Geometry check sheet. Reference: the model listing, model coordinates, mm. Face numbers are marked on the shaded views. A direction names the side the tool comes from. Round coordinates to 2 decimals unless told otherwise and drop trailing zeros. Loops run counter-clockwise (first coordinate to the right, second up) from the corner with the lowest first, then second, coordinate; pieces in that order, holes last. Notation, with made-up numbers: (41, 17) - (73, 17) arc R15 cw to (73, 27) - close; hole circle Ø1 at (79.25, 52.5). An arc over 180 degrees is marked (long way). Answer in a Markdown table with one row per item. Add a question column.
```python
from build123d import *
from build123d.topology import SkipClean

# Parameters (mm, degrees)
SKETCH_1_W                     = 41
SKETCH_1_H                     = 50
EXTRUDE_1_DEPTH                = 3
SKETCH_3_W                     = 15.5
SKETCH_3_H                     = 22
CUT_EXTRUDE_1_DEPTH            = 18
HOLE_WIZARD_M3_5_1_D           = 3.15
HOLE_WIZARD_M3_5_1_CSINK_D     = 3.55
HOLE_WIZARD_M3_5_1_CSINK_ANGLE = 90
SKETCH_16_W                    = 41
SKETCH_16_H                    = 0.872109694
EXTRUDE_5_DEPTH                = 20
SKETCH_17_W                    = 41
SKETCH_17_H                    = 50
SKETCH_17_R                    = 1.575
EXTRUDE_6_DEPTH                = 3
SKETCH_20_W                    = 26
SKETCH_20_H                    = 50
EXTRUDE_8_DEPTH                = 2
SKETCH_21_W                    = 12
SKETCH_21_H                    = 25
CUT_EXTRUDE_2_DEPTH            = 2
SKETCH_22_W                    = 26
SKETCH_22_H                    = 50
EXTRUDE_9_DEPTH                = 2
SKETCH_27_W                    = 20
SKETCH_27_H                    = 25
CUT_EXTRUDE_3_DEPTH            = 2
HOLE_WIZARD_M3_5_2_D           = 2.9
HOLE_WIZARD_M3_5_2_DEPTH       = 10
HOLE_WIZARD_M3_5_2_CSINK_D     = 3.55
HOLE_WIZARD_M3_5_2_CSINK_ANGLE = 90
HOLE_WIZARD_M3_5_2_TIP         = 0.871247898
SKETCH_36_R                    = 2.218303603
SKETCH_36_R_2                  = 1.575
SKETCH_36_R_3                  = 2.18160311
SKETCH_36_R_4                  = 2.164555566
SKETCH_36_R_5                  = 1.714538104
EXTRUDE_10_DEPTH               = 1
EXTRUDE_START                  = 1
SKETCH_37_R                    = 2.094490393
SKETCH_37_R_2                  = 1.575
SKETCH_37_R_3                  = 1.99590809
SKETCH_37_R_4                  = 2.064181582
EXTRUDE_11_DEPTH               = 1
SKETCH_38_R                    = 2.007165216
SKETCH_38_R_2                  = 1.775
SKETCH_38_R_3                  = 2.052187766
SKETCH_38_R_4                  = 2.157504148
SKETCH_38_R_5                  = 2.13214376
EXTRUDE_12_DEPTH               = 0.5


with BuildPart() as part:
    # Sketch 1 → Extrude 1 (new body)
    with BuildSketch(Plane.XY):
        Rectangle(SKETCH_1_W, SKETCH_1_H)
    extrude(amount=EXTRUDE_1_DEPTH)

    # Sketch 3 → Cut-Extrude 1 (cut)
    with BuildSketch(Plane.XY.offset(3)):
        with Locations((0, 14)):
            Rectangle(SKETCH_3_W, SKETCH_3_H)
    extrude(amount=-CUT_EXTRUDE_1_DEPTH, mode=Mode.SUBTRACT)

    # Hole Wizard M3.5 _ _1 (through all)
    with Locations(Plane.XY.offset(3)):
        with Locations((-3.5, -19), (3.5, -19), (-15.5, -11)):
            CounterSinkHole(HOLE_WIZARD_M3_5_1_D / 2, HOLE_WIZARD_M3_5_1_CSINK_D / 2, counter_sink_angle=HOLE_WIZARD_M3_5_1_CSINK_ANGLE)

    # Sketch 16 → Extrude 5 (add)
    with BuildSketch(Plane(origin=(0, 0, 0), x_dir=(-1, 0, 0), z_dir=(0, 0, -1))):
        with Locations((0, -24.563945153)):
            Rectangle(SKETCH_16_W, SKETCH_16_H)
    extrude(amount=EXTRUDE_5_DEPTH)



with BuildPart() as body_2:
    # Sketch 17 → Extrude 6 (new body)
    with BuildSketch(Plane(origin=(0, 0, -20), x_dir=(-1, 0, 0), z_dir=(0, 0, -1))):
        Rectangle(SKETCH_17_W, SKETCH_17_H)
        with Locations(Location((15.5, -11, 0), (0, 0, 180))):
            Circle(SKETCH_17_R, mode=Mode.SUBTRACT)
        with Locations(Location((3.5, -19, 0), (0, 0, 180))):
            Circle(SKETCH_17_R, mode=Mode.SUBTRACT)
        with Locations(Location((-3.5, -19, 0), (0, 0, 180))):
            Circle(SKETCH_17_R, mode=Mode.SUBTRACT)
    extrude(amount=EXTRUDE_6_DEPTH)


with BuildPart() as part_1:
    add(part.part)

    add(body_2.part)  # Extrude 8 merges body 2
    # Sketch 20 → Extrude 8 (add)
    with BuildSketch(Plane(origin=(20.5, 0, 0), x_dir=(0, 0, -1), z_dir=(1, 0, 0))):
        with Locations((10, 0)):
            Rectangle(SKETCH_20_W, SKETCH_20_H)
    extrude(amount=EXTRUDE_8_DEPTH)

    # Sketch 21 → Cut-Extrude 2 (cut)
    with BuildSketch(Plane(origin=(22.5, 0, 0), x_dir=(0, 0, -1), z_dir=(1, 0, 0))):
        with Locations((6, 12.5)):
            Rectangle(SKETCH_21_W, SKETCH_21_H)
    extrude(amount=-CUT_EXTRUDE_2_DEPTH, mode=Mode.SUBTRACT)

    # Sketch 22 → Extrude 9 (add)
    with BuildSketch(Plane.ZY.offset(20.5)):
        with Locations((-10, 0)):
            Rectangle(SKETCH_22_W, SKETCH_22_H)
    extrude(amount=EXTRUDE_9_DEPTH)

    # Sketch 27 → Cut-Extrude 3 (cut)
    with BuildSketch(Plane.ZY.offset(22.5)):
        with Locations((-10, 12.5)):
            Rectangle(SKETCH_27_W, SKETCH_27_H)
    extrude(amount=-CUT_EXTRUDE_3_DEPTH, mode=Mode.SUBTRACT)

    # Hole Wizard M3.5 _ _2
    with Locations(Plane(origin=(0, -24.127890306, 0), x_dir=(1, 0, 0), z_dir=(0, 1, 0))):
        with Locations((-18.161355758, 16.900474402), (18.309727807, 16.900474402), (-18.161355758, 2.984453016), (18.309727807, 2.984453016)):
            CounterSinkHole(HOLE_WIZARD_M3_5_2_D / 2, HOLE_WIZARD_M3_5_2_CSINK_D / 2, depth=HOLE_WIZARD_M3_5_2_DEPTH, counter_sink_angle=HOLE_WIZARD_M3_5_2_CSINK_ANGLE)
            with Locations((0, 0, -(HOLE_WIZARD_M3_5_2_DEPTH + HOLE_WIZARD_M3_5_2_TIP / 2))):  # 118° drill point
                Cone(0, HOLE_WIZARD_M3_5_2_D / 2, HOLE_WIZARD_M3_5_2_TIP, mode=Mode.SUBTRACT)

    # Sketch 36 → Extrude 10 (add)
    # profile 1 of 3: a face of its own
    with SkipClean():  # the faces are left unmerged after this step: merging them gives an invalid solid
        with BuildSketch(Plane(origin=(0, 0, 0), x_dir=(-1, 0, 0), z_dir=(0, 0, -1))):
            with Locations(Location((-3.5, -19, 0), (0, 0, 180))):
                Circle(SKETCH_36_R)
            with Locations(Location((-3.5, -19, 0), (0, 0, 180))):
                Circle(SKETCH_36_R_2, mode=Mode.SUBTRACT)
        # profile 2 of 3: a face of its own
        with BuildSketch(Plane(origin=(0, 0, 0), x_dir=(-1, 0, 0), z_dir=(0, 0, -1))):
            with Locations(Location((3.5, -19, 0), (0, 0, 180))):
                Circle(SKETCH_36_R_3)
            with Locations(Location((3.5, -19, 0), (0, 0, 180))):
                Circle(SKETCH_36_R_2, mode=Mode.SUBTRACT)
        # profile 3 of 3: a face of its own
        with BuildSketch(Plane(origin=(0, 0, 0), x_dir=(-1, 0, 0), z_dir=(0, 0, -1))):
            with Locations(Location((15.5, -11, 0), (0, 0, 180))):
                Circle(SKETCH_36_R_4)
            with Locations(Location((15.5, -10.860461896, 0), (0, 0, 270))):
                Circle(SKETCH_36_R_5, mode=Mode.SUBTRACT)
        extrude(amount=EXTRUDE_10_DEPTH)
    add(part_1.part.scale(1), mode=Mode.REPLACE)  # the faces are merged on a copy

    # Sketch 37 → Extrude 11 (add)
    # profile 1 of 3: a face of its own
    with BuildSketch(Plane.XY.offset(-20).offset(EXTRUDE_START)):
        with Locations(Location((-15.5, -11, 0), (0, 0, 180))):
            Circle(SKETCH_37_R)
        with Locations((-15.5, -11)):
            Circle(SKETCH_37_R_2, mode=Mode.SUBTRACT)
    # profile 2 of 3: a face of its own
    with BuildSketch(Plane.XY.offset(-20).offset(EXTRUDE_START)):
        with Locations(Location((-3.5, -19, 0), (0, 0, 180))):
            Circle(SKETCH_37_R_3)
        with Locations((-3.5, -19)):
            Circle(SKETCH_37_R_2, mode=Mode.SUBTRACT)
    # profile 3 of 3: a face of its own
    with BuildSketch(Plane.XY.offset(-20).offset(EXTRUDE_START)):
        with Locations(Location((3.5, -19, 0), (0, 0, 180))):
            Circle(SKETCH_37_R_4)
        with Locations((3.5, -19)):
            Circle(SKETCH_37_R_2, mode=Mode.SUBTRACT)
    extrude(amount=-EXTRUDE_11_DEPTH)

    # Sketch 38 → Extrude 12 (add)
    # profile 1 of 4: a face of its own
    with BuildSketch(Plane(origin=(0, -24.127890306, 0), x_dir=(1, 0, 0), z_dir=(0, 1, 0))):
        with Locations(Location((18.309727807, 16.900474402, 0), (0, 0, 90))):
            Circle(SKETCH_38_R)
        with Locations(Location((18.309727807, 16.900474402, 0), (0, 0, 270))):
            Circle(SKETCH_38_R_2, mode=Mode.SUBTRACT)
    # profile 2 of 4: a face of its own
    with BuildSketch(Plane(origin=(0, -24.127890306, 0), x_dir=(1, 0, 0), z_dir=(0, 1, 0))):
        with Locations(Location((18.309727807, 2.984453016, 0), (0, 0, 90))):
            Circle(SKETCH_38_R_3)
        with Locations(Location((18.309727807, 2.984453016, 0), (0, 0, 270))):
            Circle(SKETCH_38_R_2, mode=Mode.SUBTRACT)
    # profile 3 of 4: a face of its own
    with BuildSketch(Plane(origin=(0, -24.127890306, 0), x_dir=(1, 0, 0), z_dir=(0, 1, 0))):
        with Locations(Location((-18.161355758, 16.900474402, 0), (0, 0, 90))):
            Circle(SKETCH_38_R_4)
        with Locations(Location((-18.161355758, 16.900474402, 0), (0, 0, 270))):
            Circle(SKETCH_38_R_2, mode=Mode.SUBTRACT)
    # profile 4 of 4: a face of its own
    with BuildSketch(Plane(origin=(0, -24.127890306, 0), x_dir=(1, 0, 0), z_dir=(0, 1, 0))):
        with Locations(Location((-18.161355758, 2.984453016, 0), (0, 0, 90))):
            Circle(SKETCH_38_R_5)
        with Locations(Location((-18.161355758, 2.984453016, 0), (0, 0, 270))):
            Circle(SKETCH_38_R_2, mode=Mode.SUBTRACT)
    extrude(amount=EXTRUDE_12_DEPTH)


solid = part_1.part
```
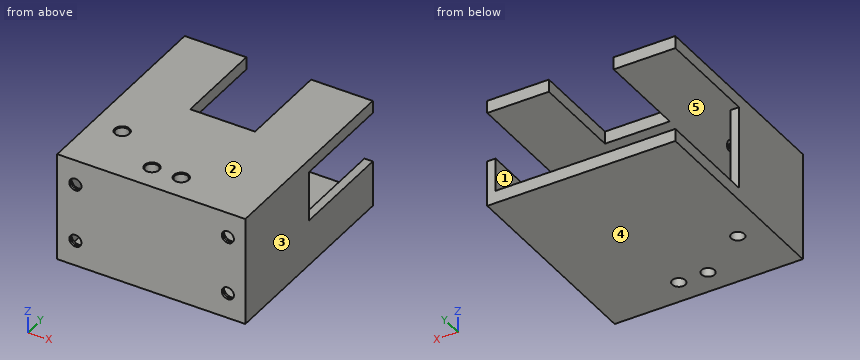
Q1. Cross-section at A-A, the plane x = -3.5. Enter the section's corners in (y, z) (3 decimals).
Q2. Depth check by flat-ended pin: P1, Ø4, axis at x = -18.16, z = -16.9, coming from the +Y side; P2, Ø2, axis at x = 1.5, z = -15, coming from the +Y side; P3, Ø1.2, axis at x = -4.5, y = -18.5, coming from the +Z side. Enter the tip coordinate at first touch or a pass-through.
Q3. Cross-section at C-C, the plane y = 10. Enter the section's corners in (x, z), plus the area to 4 significant figures.
Q4. Release check for a two-part mould opening along X. For the marked faces 3, 4 and 5 record: +X half, -X half, draft (parallel to the pull), parting line (faces both ways), or undercut.
Q5. Set-up check for the marked faces 1 and 2: record each of +Z, -Z, +X, -X, +Y, -Y from which the full face is reachable in a straight line by a thin tool's end or side.
Q6. Cross-section at B-B, the plane y = 1.5. Enter the section's corners in (x, z), plus the area to 3 significant figures.
Q7. Cross-section at D-D, the plane x = 9.5. Enter the section's corners in (y, z).
Q8. Scan lines: line 1 (Y direction, x = -15.5, z = -19.55) (1 decimal); line 2 (Y direction, x = -15.5, z = -0.35) (3 decimals); line 3 (Z direction, x = 14, y = -11). Record each from-to range of solid material in increasing order. Write a range as from..to.
Check sheet entries:
| question | item | result |
|---|---|---|
| 1 | outline | (-25, -23) - (-20.575, -23) - (-20.575, -19) - (-20.996, -19) - (-20.996, -20) - (-24.128, -20) - (-24.128, 0) - (-21.182, 0) - (-21.182, -1) - (-20.575, -1) - (-20.575, 2.8) - (-20.775, 3) - (-25, 3) - close; (-17.425, -23) - (25, -23) - (25, -20) - (-17.004, -20) - (-17.004, -19) - (-17.425, -19) - close; (-17.425, -1) - (-16.818, -1) - (-16.818, 0) - (3, 0) - (3, 3) - (-17.225, 3) - (-17.425, 2.8) - close |
| 2 | P1 | y = -23.63 |
| 2 | P2 | y = -24.13 |
| 2 | P3 | z = 2.94 |
| 3 | outline | (-22.5, -23) - (22.5, -23) - (22.5, -12) - (20.5, -12) - (20.5, -20) - (-22.5, -20) - close; (-22.5, 0) - (-7.75, 0) - (-7.75, 3) - (-22.5, 3) - close; (7.75, 0) - (22.5, 0) - (22.5, 3) - (7.75, 3) - close |
| 3 | area | 239.5 mm² |
| 4 | face 3 | +X half |
| 4 | face 4 | draft |
| 4 | face 5 | undercut |
| 5 | face 1 | +Y |
| 5 | face 2 | +Z, +X, -X, +Y, -Y |
| 6 | outline | (-22.5, -23) - (22.5, -23) - (22.5, -12) - (20.5, -12) - (20.5, -20) - (-22.5, -20) - close; (-22.5, 0) - (22.5, 0) - (22.5, 3) - (-22.5, 3) - close |
| 6 | area | 286 mm² |
| 7 | outline | (-25, -23) - (25, -23) - (25, -20) - (-24.13, -20) - (-24.13, 0) - (25, 0) - (25, 3) - (-25, 3) - close |
| 8 | line 1 | -25..-24.1, -13.1..-12.6, -9.4..-8.9 |
| 8 | line 2 | -25..-24.128, -13.165..-12.575, -9.146..-8.835 |
| 8 | line 3 | -23..-20, 0..3 |
